from build123d import *
from OCP.BRepFilletAPI import BRepFilletAPI_MakeChamfer

# Parameters (mm, degrees)
BOSS_EXTRUDE1_DEPTH = 15
BOSS_EXTRUDE2_DEPTH = 15
SKETCH6_W           = 115
SKETCH6_H           = 1.4
CUT_EXTRUDE2_DEPTH  = 10
CUT_EXTRUDE3_DEPTH  = 10
CUT_EXTRUDE4_DEPTH  = 10
BOSS_EXTRUDE3_DEPTH = 1
CUT_EXTRUDE5_REACH  = 117.913
SKETCH10_W          = 115
SKETCH10_H          = 5.7
SKETCH13_W          = 20.2
SKETCH13_H          = 23
CUT_EXTRUDE6_DEPTH  = 111.121977825
FILLET1_R           = 6
SKETCH14_W          = 6
SKETCH14_H          = 31
CUT_EXTRUDE7_DEPTH  = 4.5
FILLET2_R           = 3
SKETCH16_W          = 10
SKETCH16_H          = 2.5
CUT_EXTRUDE8_DEPTH  = 1.8
CHAMFER1_SIZE       = 0.5
CHAMFER1_SIZE_2     = 0.619555405
CHAMFER2_SIZE       = 1
CHAMFER3_SIZE       = 5
CHAMFER3_SIZE2      = 1.339745962
CUT_EXTRUDE12_REACH = 112.118
CHAMFER4_SIZE       = 0.2
CHAMFER4_SIZE_2     = 0.141421356
SKETCH25_W          = 6
SKETCH25_H          = 12
BOSS_EXTRUDE6_DEPTH = 15
FILLET4_START       = -1
FILLET4_DEPTH       = 16
FILLET4_2_DEPTH     = 15
CUT_EXTRUDE15_DEPTH = 15
CUT_EXTRUDE16_DEPTH = 10
CHAMFER5_SIZE       = 0.5
CHAMFER5_SIZE2      = 0.353553391
CHAMFER6_SIZE       = 0.65
SKETCH29_W          = 10
SKETCH29_H          = 0.8
CUT_EXTRUDE17_DEPTH = 3.2


with BuildPart() as part:
    # Sketch3 → Boss-Extrude1 (new body)
    with BuildSketch(Plane.XY):
        Polygon((0, 0), (0, 20.2), (-20.2, 20.2), (-20.2, -10.8), (-26.2, -10.8), (-26.2, 49.2), (-69.1, 49.2), (-69.1, 55.2), (5.9, 55.2), (65.9, 55.2), (65.9, 45.2), (6, 45.2), (6, 0), align=None)
    extrude(amount=BOSS_EXTRUDE1_DEPTH)

    # Sketch4 → Boss-Extrude2 (add)
    with BuildSketch(Plane.XY.offset(15)):
        with BuildLine():
            Line((-88.1, 30.2), (-94.1, 30.2))
            ThreePointArc((-94.1, 30.2), (-86.77766953, 47.87766953), (-69.1, 55.2))
            Line((-69.1, 55.2), (-69.1, 49.2))
            ThreePointArc((-69.1, 49.2), (-82.535028843, 43.635028843), (-88.1, 30.2))
        make_face()
    extrude(amount=-BOSS_EXTRUDE2_DEPTH)

    # Sketch6 → Cut-Extrude2 (cut)
    with BuildSketch(Plane.XY.offset(15)):
        with Locations((-11.6, 52.7)):
            Rectangle(SKETCH6_W, SKETCH6_H)
    extrude(amount=-CUT_EXTRUDE2_DEPTH, mode=Mode.SUBTRACT)

    # Sketch7 → Cut-Extrude3 (cut)
    with BuildSketch(Plane.XY.offset(15)):
        with BuildLine():
            Line((-92.3, 30.2), (-90.9, 30.2))
            ThreePointArc((-90.9, 30.2), (-84.51492783, 45.61492783), (-69.1, 52))
            Line((-69.1, 52), (-69.1, 53.4))
            ThreePointArc((-69.1, 53.4), (-85.504877324, 46.604877324), (-92.3, 30.2))
        make_face()
    extrude(amount=-CUT_EXTRUDE3_DEPTH, mode=Mode.SUBTRACT)

    # Sketch8 → Cut-Extrude4 (cut)
    with BuildSketch(Plane.XY.offset(15)):
        Polygon((45.9, 53.4), (65.9, 53.4), (65.9, 48.4), (45.9, 52), align=None)
    extrude(amount=-CUT_EXTRUDE4_DEPTH, mode=Mode.SUBTRACT)

    # Sketch9 → Boss-Extrude3 (add)
    with BuildSketch(Plane.XY.offset(15)):
        with BuildLine():
            Line((-69.1, 52), (45.9, 52))
            Line((45.9, 52), (45.9, 53.4))
            Line((45.9, 53.4), (-69.1, 53.4))
            ThreePointArc((-69.1, 53.4), (-85.504877324, 46.604877324), (-92.3, 30.2))
            Line((-92.3, 30.2), (-90.9, 30.2))
            ThreePointArc((-90.9, 30.2), (-84.51492783, 45.61492783), (-69.1, 52))
        make_face()
    extrude(amount=-BOSS_EXTRUDE3_DEPTH)

    # Cut-Extrude5: up to this face of the body (flat: up to its plane)
    cut_extrude5_end = Plane(part.part.faces().sort_by_distance((-11.6, 52, 9.5))[0])
    # Sketch10 → Cut-Extrude5 (cut, up to the picked face)
    with BuildSketch(Plane(origin=(0, 55.2, 0), x_dir=(-1, 0, 0), z_dir=(0, 1, 0)), mode=Mode.PRIVATE) as cut_extrude5_sk1:
        with Locations((11.6, 8.65)):
            Rectangle(SKETCH10_W, SKETCH10_H)
    cut_extrude5_tool1 = split(extrude(cut_extrude5_sk1.sketch, amount=-CUT_EXTRUDE5_REACH, mode=Mode.PRIVATE), bisect_by=cut_extrude5_end, keep=Keep.BOTH, mode=Mode.PRIVATE)
    add(cut_extrude5_tool1.solids().sort_by(Axis((-11.6, 55.2, 8.65), (0, -1, 0)))[0], mode=Mode.SUBTRACT)

    # Sketch13 → Cut-Extrude6 (cut, through all)
    with BuildSketch(Plane.XY.offset(15)):
        with Locations((-10.1, 37.7)):
            Rectangle(SKETCH13_W, SKETCH13_H)
    extrude(amount=-CUT_EXTRUDE6_DEPTH, mode=Mode.SUBTRACT)

    # Fillet1
    fillet1_edges = [part.edges().sort_by_distance(p)[0] for p in [
        (-20.2, 26.2, 7.5),
        (-20.2, 49.2, 7.5),
        (0, 49.2, 7.5),
        (0, 26.2, 7.5),
    ]]
    fillet(fillet1_edges, radius=FILLET1_R)

    # Sketch14 → Cut-Extrude7 (cut)
    with BuildSketch(Plane.XY.offset(15)):
        with Locations((-23.2, 4.7)):
            Rectangle(SKETCH14_W, SKETCH14_H)
    extrude(amount=-CUT_EXTRUDE7_DEPTH, mode=Mode.SUBTRACT)

    # Fillet2
    fillet2_edges = [part.edges().sort_by_distance(p)[0] for p in [
        (-26.2, 49.2, 7.5),
        (6, 45.2, 7.5),
        (-26.2, 20.2, 12.75),
        (6, 0, 7.5),
        (0, 0, 7.5),
        (-20.2, -10.8, 5.25),
        (-26.2, -10.8, 5.25),
    ]]
    fillet(fillet2_edges, radius=FILLET2_R - 0.0001)  # a hair under: the kernel refuses the full size

    # Sketch16 → Cut-Extrude8 (cut)
    with BuildSketch(Plane(origin=(0, 55.2, 0), x_dir=(-1, 0, 0), z_dir=(0, 1, 0))):
        with Locations((64.1, 12.75)):
            Rectangle(SKETCH16_W, SKETCH16_H)
    extrude(amount=-CUT_EXTRUDE8_DEPTH, mode=Mode.SUBTRACT)

    # Chamfer1
    # the kernel refuses this chamfer: 0.619555405, 0.5 mm, written as the material it takes off along each edge
    with BuildSketch(Plane(origin=(65.9, 55.2, -1.285841494), x_dir=(-1, 0, 0), z_dir=(0, 0, 1)), Plane(origin=(65.9, 45.2, -1.285841494), x_dir=(0, 1, 0), z_dir=(0, 0, 1))) as chamfer1_piece_1:
        Polygon((CHAMFER1_SIZE, 0), (0, CHAMFER1_SIZE), (0, 0), align=None)
    extrude(amount=17.571682988, mode=Mode.SUBTRACT)
    with BuildSketch(Plane(origin=(-88.1, 30.2, 16.303301327), x_dir=(-1, 0, 0), z_dir=(0, 0, -1))) as chamfer1_piece_2:
        with BuildLine():
            Line((CHAMFER1_SIZE, 0), (-0.006759226, 0.506759226))
            ThreePointArc((-0.006759226, 0.506759226), (-0.001786833, 0.26056951), (0, 0))
            Line((0, 0), (CHAMFER1_SIZE, 0))
        make_face()
    extrude(amount=17.606602654, mode=Mode.SUBTRACT)
    with BuildSketch(Plane(origin=(-94.1, 30.2, 16.285841494), x_dir=(1, 0, 0), z_dir=(0, 0, -1))) as chamfer1_piece_3:
        with BuildLine():
            Line((CHAMFER1_SIZE, 0), (0.004902903, -0.495097097))
            ThreePointArc((0.004902903, -0.495097097), (0.001296043, -0.254559377), (0, 0))
            Line((0, 0), (CHAMFER1_SIZE, 0))
        make_face()
    extrude(amount=17.571682988, mode=Mode.SUBTRACT)
    with BuildSketch(Plane(origin=(65.9, 53.4, 16.285841494), x_dir=(-1, 0, 0), z_dir=(0, 0, -1))) as chamfer1_piece_4:
        Polygon((CHAMFER1_SIZE, 0), (0, CHAMFER1_SIZE), (0, 0), align=None)
    extrude(amount=11.285841494, mode=Mode.SUBTRACT)
    with BuildSketch(Plane(origin=(65.9, 48.4, 16.600156341), x_dir=(-0.9841833239736955, 0.17715299831526463, 0), z_dir=(0, 0, -1))) as chamfer1_piece_5:
        Polygon((CHAMFER1_SIZE, 0), (-CHAMFER1_SIZE_2 * 0.177152998223, -CHAMFER1_SIZE_2 * 0.984183323461), (0, 0), align=None)
    extrude(amount=11.600156341, mode=Mode.SUBTRACT)

    # Chamfer2
    chamfer2_edges = [part.edges().sort_by_distance(p)[0] for p in [
        (-10.1, 49.2, 15),
        (-10.1, 49.2, 0),
        (0, 37.7, 15),
        (0, 37.7, 0),
        (-10.1, 26.2, 15),
        (-10.1, 26.2, 0),
        (-20.2, 37.7, 15),
        (-20.2, 37.7, 0),
        (-1.757359313, 47.442640687, 15),
        (-1.757359313, 47.442640687, 0),
        (-1.757359313, 27.957359313, 15),
        (-1.757359313, 27.957359313, 0),
        (-18.442640687, 27.957359313, 15),
        (-18.442640687, 27.957359313, 0),
        (-18.442640687, 47.442640687, 15),
        (-18.442640687, 47.442640687, 0),
    ]]
    chamfer(chamfer2_edges, length=CHAMFER2_SIZE)

    # Chamfer3
    chamfer3_edges = [part.edges().sort_by_distance(p)[0] for p in [
        (45.9, 55.2, 8.65),
    ]]
    chamfer3_side = [part.faces().sort_by_distance(p)[0] for p in [
        (64.046661535, 55.2, 7.5),
    ]]
    chamfer(chamfer3_edges, length=CHAMFER3_SIZE, length2=CHAMFER3_SIZE2, reference=chamfer3_side[0])

    # Cut-Extrude12: up to this face of the body (flat: up to its plane)
    cut_extrude12_end = Plane(part.part.faces().sort_by_distance((-5.656799941, 54.307895333, 11.5))[0])
    # Sketch20 → Cut-Extrude12 (cut, up to the picked face)
    with BuildSketch(Plane.XY.offset(15), mode=Mode.PRIVATE) as cut_extrude12_sk1:
        Polygon((45.9, 52), (42.7, 55.2), (44.1, 55.2), (45.9, 53.4), align=None)
    cut_extrude12_tool1 = split(extrude(cut_extrude12_sk1.sketch, amount=-CUT_EXTRUDE12_REACH, mode=Mode.PRIVATE), bisect_by=cut_extrude12_end, keep=Keep.BOTH, mode=Mode.PRIVATE)
    add(cut_extrude12_tool1.solids().sort_by(Axis((44.617333, 53.917333, 15), (0, 0, -1)))[0], mode=Mode.SUBTRACT)

    # Chamfer4
    # the kernel refuses this chamfer: 0.2, 0.141421356 mm, written as the material it takes off along each edge
    with BuildSketch(Plane(origin=(44.5, 53.4, 10.985663402), x_dir=(-0.7071067811865476, 0.7071067811865476, 0), z_dir=(0, 0, 1))) as chamfer4_piece_1:
        Polygon((CHAMFER4_SIZE, 0), (CHAMFER4_SIZE_2 * 0.707106782373, CHAMFER4_SIZE_2 * 0.707106782373), (0, 0), align=None)
    extrude(amount=3.014336598, mode=Mode.SUBTRACT)
    with BuildSketch(Plane(origin=(44.1, 55.2, 15.514336598), x_dir=(1, 0, 0), z_dir=(0, 0, -1))) as chamfer4_piece_2:
        Polygon((CHAMFER4_SIZE_2 * 1.00000000168, 0), (CHAMFER4_SIZE * 0.707106781187, CHAMFER4_SIZE * 0.707106781186), (0, 0), align=None)
    extrude(amount=4.528673195, mode=Mode.SUBTRACT)

    # Sketch25 → Boss-Extrude6 (add)
    with BuildSketch(Plane.XY.offset(15)):
        with Locations((9, 26.1)):
            Rectangle(SKETCH25_W, SKETCH25_H)
    extrude(amount=-BOSS_EXTRUDE6_DEPTH)

    # Fillet4: read off the stored shape, not the designer's step
    # Fillet4 outline → Fillet4 (cut)
    with BuildSketch(Plane.XY.offset(FILLET4_START)):
        with BuildLine():
            ThreePointArc((9, 32.1), (11.121320344, 31.221320344), (12, 29.1))
            Line((12, 29.1), (12, 32.1))
            Line((12, 32.1), (9, 32.1))
        make_face()
        with BuildLine():
            ThreePointArc((12, 23.1), (11.121320344, 20.978679656), (9, 20.1))
            Line((9, 20.1), (12, 20.1))
            Line((12, 20.1), (12, 23.1))
        make_face()
    extrude(amount=FILLET4_DEPTH, mode=Mode.SUBTRACT)

    # Fillet4 2 outline → Fillet4 2 (add)
    with BuildSketch(Plane.XY):
        with BuildLine():
            Line((6, 32.1), (9, 32.1))
            ThreePointArc((9, 32.1), (6.878679656, 32.978679656), (6, 35.1))
            Line((6, 35.1), (6, 32.1))
        make_face()
        with BuildLine():
            ThreePointArc((6, 17.1), (6.878679656, 19.221320344), (9, 20.1))
            Line((9, 20.1), (6, 20.1))
            Line((6, 20.1), (6, 17.1))
        make_face()
    extrude(amount=FILLET4_2_DEPTH)

    # Sketch26 → Cut-Extrude15 (cut)
    with BuildSketch(Plane.XY.offset(15)):
        Polygon((12, 29.1), (10, 29.1), (7.402667467, 31.1), (6, 31.1), (6, 21.1), (8.459958458, 21.1), (10, 23.1), (12, 23.1), align=None)
    extrude(amount=-CUT_EXTRUDE15_DEPTH, mode=Mode.SUBTRACT)

    # Sketch27 → Cut-Extrude16 (cut)
    with BuildSketch(Plane.XY.offset(15)):
        Polygon((62.9, 53.4), (61.1, 55.2), (62.1, 55.2), (63.9, 53.4), align=None)
    extrude(amount=-CUT_EXTRUDE16_DEPTH, mode=Mode.SUBTRACT)

    # Chamfer5: one chamfer whose edges measure the first distance from different faces: ONE call of the kernel's chamfer builder (chamfer() names one face for all edges)
    chamfer5_edges_1 = [part.edges().sort_by_distance(p)[0] for p in [
        (62.9, 53.4, 10),
    ]]
    chamfer5_side_1 = [part.faces().sort_by_distance(p)[0] for p in [
        (62, 54.3, 10),
    ]]
    chamfer5_edges_2 = [part.edges().sort_by_distance(p)[0] for p in [
        (62.1, 55.2, 10),
    ]]
    chamfer5_side_2 = [part.faces().sort_by_distance(p)[0] for p in [
        (63, 54.3, 10),
    ]]
    chamfer5 = BRepFilletAPI_MakeChamfer(part.part.solid().wrapped)
    for e in chamfer5_edges_1:
        chamfer5.Add(CHAMFER5_SIZE, CHAMFER5_SIZE2, e.wrapped, chamfer5_side_1[0].wrapped)  # the first distance lies on this face
    for e in chamfer5_edges_2:
        chamfer5.Add(CHAMFER5_SIZE, CHAMFER5_SIZE2, e.wrapped, chamfer5_side_2[0].wrapped)  # the first distance lies on this face
    add(Compound.cast(chamfer5.Shape()), mode=Mode.REPLACE)

    # Chamfer6
    chamfer6_edges = [part.edges().sort_by_distance(p)[0] for p in [
        (-84.51492783, 45.61492783, 14),
        (-85.504877324, 46.604877324, 14),
        (-11.6, 52, 14),
        (-7.370710678, 53.4, 14),
    ]]
    chamfer(chamfer6_edges, length=CHAMFER6_SIZE)

    # Sketch29 → Cut-Extrude17 (cut)
    with BuildSketch(Plane(origin=(0, 55.2, 0), x_dir=(-1, 0, 0), z_dir=(0, 1, 0))):
        with Locations((-40.9, 5.4)):
            Rectangle(SKETCH29_W, SKETCH29_H)
    extrude(amount=-CUT_EXTRUDE17_DEPTH, mode=Mode.SUBTRACT)


solid = part.part
Could you check a few things on this model? Use its own coordinates, in mm. A direction names the side the tool comes from. Round coordinates to 2 decimals unless told otherwise and drop trailing zeros. Loops run counter-clockwise (first coordinate to the right, second up) from the corner with the lowest first, then second, coordinate; pieces in that order, holes last. Notation, with made-up numbers: (2, 55) - (25, 55) arc R19 cw to (25, 63) - close; hole circle Ø4 at (40, -5). An arc over 180 degrees is marked (long way). Write item = value, one per line.
1) Imagine slicing it at A-A (y = 6). Please give me the cut outline in (x, z).
Computed:
outline = (-26.2, 0) - (-20.2, 0) - (-20.2, 10.5) - (-26.2, 10.5) - close; (0, 0) - (6, 0) - (6, 15) - (0, 15) - close
2) On a 3-axis mill with a long thin cutter (end or side, diameter ignored), from which of +Z, -Z, +X, -X, +Y, -Y can I reach the whole of each face in a straight line? I mean faces 5 (the flat face through (-20.2, 38, 8)), 6 (the cylindrical face through (-27.06, 48.3, 7.6)), 7 (the conical face through (-1.683, 27.787, 0.826)). Say none if no direction works.
Computed:
face_5 = +Z, -Z
face_6 = +Z, -Z, -Y
face_7 = -Z
3) I need wall thicknesses on line 1 along X through (y, z) = (45.5, 10.25); line 2 along Y through (x, z) = (-57, 5.5); line 3 along X through (y, z) = (42.5, 12.5). Which ranges of each line are inside material? Lowest first, please. Write a range as from..to.
Computed:
line_1 = -88.87..-86.54, -84.63..-80.37, -26.2..-19.74, -0.46..65.7
line_2 = 49.2..52, 53.4..55.2
line_3 = -90.86..-88.77, -87.1..-83.58, -26.2..-20.2, 0..6.02
4) Imagine slicing it at C-C (x = 14). Please give me the cut outline in (y, z).
Computed:
outline = (45.2, 0) - (55.2, 0) - (55.2, 5.8) - (53.4, 5.8) - (53.4, 5) - (52, 5) - (52, 13.35) - (52.65, 14) - (52.75, 14) - (53.4, 13.35) - (53.4, 11.5) - (55.2, 11.5) - (55.2, 15) - (45.2, 15) - close
5) Imagine slicing it at B-B (x = -12.5). Please give me the cut outline in (y, z).
Computed:
outline = (20.2, 0) - (25.2, 0) - (26.2, 1) - (26.2, 14) - (25.2, 15) - (20.2, 15) - close; (49.2, 1) - (50.2, 0) - (55.2, 0) - (55.2, 5.8) - (53.4, 5.8) - (53.4, 5) - (52, 5) - (52, 13.35) - (52.65, 14) - (52.75, 14) - (53.4, 13.35) - (53.4, 11.5) - (55.2, 11.5) - (55.2, 15) - (50.2, 15) - (49.2, 14) - close
6) Imagine slicing it at D-D (z = 8). Give the number of separate pieces and of enclosed holes in the cut face, and give its area (3 significant figures).
Computed:
separate_pieces = 4
enclosed_holes = 1
area = 1,600 mm2
7) If we mould it in two halves opening along X, with no side actions, what happens to faces 1 (the flat face through (55.79, 50.22, 10.07)), 2 (the flat face through (-12, 55.2, 13)), 3 (the conical face through (-18.517, 47.613, 0.826)), 4 (the cylindrical face through (-86.795, 47.861, 7.605))? For each: pulls with the +X half, pulls with the -X half, needs draft (parallel to the pull), parting line crosses it, or undercut.
Computed:
face_1 = pulls with the +X half
face_2 = needs draft
face_3 = undercut
face_4 = pulls with the -X half
8) I'm going to push flat-ended pins straight in: P1, Ø3, axis at x = -24, y = 2.5, coming from the +Z side; P2, Ø6, axis at y = -4, z = 5.5, coming from the -X side; P3, Ø7.5, axis at x = 48, z = 9, coming from the -Y side. Where does each tip first touch, or does it pass through?
Computed:
P1 = 10.5
P2 = -26.2
P3 = 45.2
